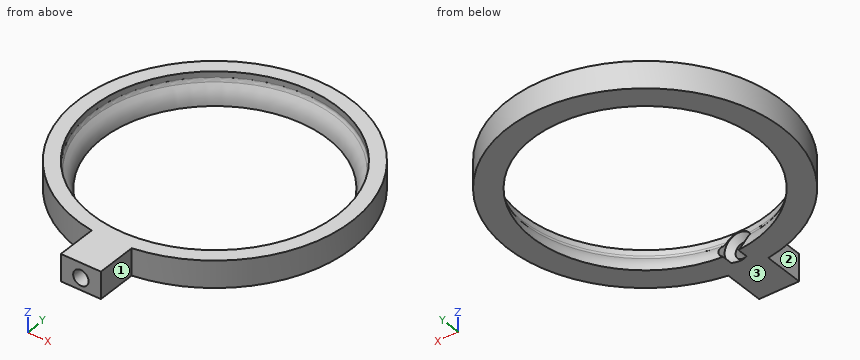
```python
from build123d import *

# Parameters (mm, degrees)
SKETCH002_W = 7
SKETCH002_H = 14.789333
PAD_DEPTH   = 9.367216


with BuildPart() as part:
    # Sketch → Revolution (revolve)
    with BuildSketch(Plane.XZ):
        with BuildLine():
            ThreePointArc((42.295694, 49.859657), (40.314757, 47.066424), (39.35, 43.780773))
            Line((47.827152, 43.780773), (39.35, 43.780773))
            Line((47.827152, 53.147989), (47.827152, 43.780773))
            Line((42.827152, 53.147989), (47.827152, 53.147989))
            Line((42.827152, 51.147989), (42.827152, 53.147989))
            ThreePointArc((42.295694, 49.859657), (42.68907, 50.451166), (42.827152, 51.147989))
        make_face()
    revolve(axis=Axis((0, 0, 0), (0, 0, 1)))

    # Sketch002 (on DatumPlane) → Pad (new body)
    with BuildSketch(Plane(origin=(0, 0, 43.780773), x_dir=(-1, 0, 0), z_dir=(0, 0, 1))):
        with Locations((-3.5, 54.037153)):
            Rectangle(SKETCH002_W, SKETCH002_H)
    pad = extrude(amount=PAD_DEPTH)

    # Mirrored: Pad across Sketch002 V_Axis
    add(pad.mirror(Plane(origin=(0, 0, 43.780773), x_dir=(0, 0, 1), z_dir=(-1, 0, 0))))

    # Sketch003 → Groove (revolve, cut)
    with BuildSketch(Plane(origin=(0, -43, 48), x_dir=(0, 1, 0), z_dir=(1, 0, 0))):
        Polygon((0, 5), (-2, 2.693579), (-42.222773, 2.693579), (-42.408872, 0), (36.192486, 0), (36.192486, 5), align=None)
    revolve(axis=Axis((0, -43, 48), (0, 1, 0)), mode=Mode.SUBTRACT)


solid = part.part
```
Model file for the job. Use its own axes, mm. Face numbers are marked on the shaded views. A direction names the side the tool comes from. Round coordinates to 2 decimals unless told otherwise and drop trailing zeros. Write each loop counter-clockwise with the first axis right and the second up, starting at its lowest first coordinate (ties: lowest second). Pieces come first, ordered by that corner, then holes. Notation, with made-up numbers: M -11.5,62 L 6.5,62 A14 ccw 6.5,66 Z; hole C 67.5,14.5 d7. An arc over 180 degrees is marked long. Put each result on its own line as item: value.
Item 1: Cut at A-A (y = 0). List the corners of the cut face in (x, z).
Responses:
outline: M -47.83,43.78 L -39.35,43.78 A10.38 ccw -42.3,49.86 A1.83 cw -42.83,51.15 L -42.83,53.15 L -47.83,53.15 Z; M 39.35,43.78 L 47.83,43.78 L 47.83,53.15 L 42.83,53.15 L 42.83,51.15 A1.83 cw 42.3,49.86 A10.38 ccw Z
Item 2: Cut at B-B (x = 0). List the corners of the cut face in (y, z).
Responses:
outline: M -61.43,43.78 L -43.68,43.78 L -45,45.31 L -61.43,45.31 Z; M -61.43,50.69 L -45,50.69 L -43,53 L -42.83,53 L -42.83,53.15 L -61.43,53.15 Z; M 39.35,43.78 L 47.83,43.78 L 47.83,53.15 L 42.83,53.15 L 42.83,51.15 A1.83 cw 42.3,49.86 A10.38 ccw Z
Item 3: Tool access for the marked faces 1, 2 and 3: list every direction of +Z, -Z, +X, -X, +Y, -Y with a clear straight run to the whole face (end or side of a thin tool).
Responses:
face 1: +Z, -Z, +X, -Y
face 2: +Z, -Z, -X, -Y
face 3: -Z, +X, -X, +Y, -Y
Item 4: Flat gauge pins, fed straight in: P1, Ø3, axis at y = -58, z = 48.5, coming from the +X side; P2, Ø5, axis at x = -36.5, z = 47, coming from the +Y side; P3, Ø4, axis at x = -23, z = 48.5, coming from the +Y side. Where does each tip first touch, or does it go through?
Responses:
P1: x = 7
P2: y = 33.64
P3: y = 42.97
Item 5: Probe L1, parallel to X at y = -49.5, z = 48; L2, parallel to X at y = 0, z = 52; L3, parallel to Z at x = 0, y = -48. List the from-to ranges inside material, lowest first. Write a range as from..to.
Responses:
L1: -7..-2.69, 2.69..7
L2: -47.83..-42.83, 42.83..47.83
L3: 43.78..45.31, 50.69..53.15
Item 6: Cut at C-C (z = 48). List the corners of the cut face in (x, y).
Responses:
outline: M -7,-61.43 L -2.69,-61.43 L -2.69,-45 L -5,-43 L -5,-40.52 A40.83 cw long 5,-40.52 L 5,-43 L 2.69,-45 L 2.69,-61.43 L 7,-61.43 L 7,-47.31 A47.83 ccw long -7,-47.31 Z
